```python
from build123d import *

# Parameters (mm, degrees)
BOSS_EXTRUDE1_OUTLINE_R = 7.5
BOSS_EXTRUDE1_DEPTH     = 30
SKETCH1_3_R             = 7.5
SKETCH1_3_R_2           = 5
BOSS_EXTRUDE2_DEPTH     = 5
FILLET1_R               = 10
CUT_EXTRUDE6_DEPTH      = 4
SKETCH5_3_R             = 2
CUT_EXTRUDE7_DEPTH      = 35
SKETCH10_R              = 1.5
CUT_EXTRUDE11_DEPTH     = 4
CUT_EXTRUDE12_START     = -2.5
SKETCH10_5_R            = 1.5
CUT_EXTRUDE12_DEPTH     = 2.5
CUT_EXTRUDE13_DEPTH     = 34


# Read off the part's stored shape, not the designer's step: Boss-Extrude1
with BuildPart() as part:
    # Boss-Extrude1 outline → Boss-Extrude1 (new body)
    with BuildSketch(Plane(origin=(0, 0, 0), x_dir=(1, 0, 0), z_dir=(0, 1, 0))):
        Polygon((-33.5, 13), (-33.5, -13), (-15, -13), (-15, -21.5), (-2, -21.5), (-2, -10.5), (2, -10.5), (2, -21.5), (15, -21.5), (15, -13), (33.5, -13), (33.5, 13), align=None)
        with Locations((-15, 0)):
            Circle(BOSS_EXTRUDE1_OUTLINE_R, mode=Mode.SUBTRACT)
        with Locations((15, 0)):
            Circle(BOSS_EXTRUDE1_OUTLINE_R, mode=Mode.SUBTRACT)
    extrude(amount=BOSS_EXTRUDE1_DEPTH)

    # Sketch1<3> → Boss-Extrude2 (add)
    # profile 1 of 2: a face of its own
    with BuildSketch(Plane(origin=(0, 0, 0), x_dir=(1, 0, 0), z_dir=(0, 1, 0))):
        with Locations(Location((-15, 0, 0), (0, 0, 270))):
            Circle(SKETCH1_3_R)
        with Locations(Location((-15, 0, 0), (0, 0, 270))):
            Circle(SKETCH1_3_R_2, mode=Mode.SUBTRACT)
    # profile 2 of 2: a face of its own
    with BuildSketch(Plane(origin=(0, 0, 0), x_dir=(1, 0, 0), z_dir=(0, 1, 0))):
        with Locations(Location((15, 0, 0), (0, 0, 270))):
            Circle(SKETCH1_3_R)
        with Locations(Location((15, 0, 0), (0, 0, 270))):
            Circle(SKETCH1_3_R_2, mode=Mode.SUBTRACT)
    extrude(amount=BOSS_EXTRUDE2_DEPTH)

    # Fillet1
    fillet1_edges = [part.edges().sort_by_distance(p)[0] for p in [
        (-33.5, 15, -13),
        (33.5, 15, -13),
        (33.5, 15, 13),
        (-33.5, 15, 13),
    ]]
    fillet(fillet1_edges, radius=FILLET1_R)

    # Sketch5 → Cut-Extrude6 (cut)
    with BuildSketch(Plane(origin=(15, 0, 0), x_dir=(0, 0, -1), z_dir=(1, 0, 0))):
        with BuildLine():
            Line((-20.75, 17.020725942), (-20.75, 15))
            Line((-20.75, 15), (-19.25, 15))
            ThreePointArc((-19.25, 15), (-17.25, 17), (-15.25, 15))
            Line((-15.25, 15), (-13.75, 15))
            Line((-13.75, 15), (-13.75, 17.020725942))
            Line((-13.75, 17.020725942), (-17.25, 19.041451884))
            Line((-17.25, 19.041451884), (-20.75, 17.020725942))
        make_face()
        with BuildLine():
            Line((-19.25, 15), (-20.75, 15))
            Line((-20.75, 15), (-20.75, 12.979274058))
            Line((-20.75, 12.979274058), (-17.25, 10.958548116))
            Line((-17.25, 10.958548116), (-13.75, 12.979274058))
            Line((-13.75, 12.979274058), (-13.75, 15))
            Line((-13.75, 15), (-15.25, 15))
            ThreePointArc((-15.25, 15), (-17.25, 13), (-19.25, 15))
        make_face()
    extrude(amount=-CUT_EXTRUDE6_DEPTH, mode=Mode.SUBTRACT)

    # Sketch5<3> → Cut-Extrude7 (cut)
    with BuildSketch(Plane(origin=(15, 0, 0), x_dir=(0, 0, -1), z_dir=(1, 0, 0))):
        with Locations((-17.25, 15)):
            Circle(SKETCH5_3_R)
    extrude(amount=-CUT_EXTRUDE7_DEPTH, mode=Mode.SUBTRACT)

    # Sketch10 → Cut-Extrude11 (cut)
    with BuildSketch(Plane(origin=(30.5, 0, 0), x_dir=(0, 0, -1), z_dir=(1, 0, 0))):
        with Locations((0, 22)):
            Circle(SKETCH10_R)
        with Locations((0, 8)):
            Circle(SKETCH10_R)
    cut_extrude11 = extrude(amount=CUT_EXTRUDE11_DEPTH, mode=Mode.SUBTRACT)

    # Sketch10<5> → Cut-Extrude12 (cut)
    # profile 1 of 5: a face of its own
    with BuildSketch(Plane(origin=(30.5, 0, 0), x_dir=(0, 0, -1), z_dir=(1, 0, 0)).offset(CUT_EXTRUDE12_START)):
        Polygon((-2.725, 30), (2.725, 30), (2.725, 23.573279484), (0, 25.146558967), (-2.725, 23.573279484), align=None)
    # profile 2 of 5: a face of its own
    with BuildSketch(Plane(origin=(30.5, 0, 0), x_dir=(0, 0, -1), z_dir=(1, 0, 0)).offset(CUT_EXTRUDE12_START)):
        Polygon((2.725, 20.426720516), (2.725, 23.573279484), (0, 25.146558967), (-2.725, 23.573279484), (-2.725, 20.426720516), (0, 18.853441033), align=None)
        with Locations((0, 22)):
            Circle(SKETCH10_5_R, mode=Mode.SUBTRACT)
    # profile 3 of 5: a face of its own
    with BuildSketch(Plane(origin=(30.5, 0, 0), x_dir=(0, 0, -1), z_dir=(1, 0, 0)).offset(CUT_EXTRUDE12_START)):
        with Locations((0, 22)):
            Circle(SKETCH10_5_R)
    # profile 4 of 5: a face of its own
    with BuildSketch(Plane(origin=(30.5, 0, 0), x_dir=(0, 0, -1), z_dir=(1, 0, 0)).offset(CUT_EXTRUDE12_START)):
        Polygon((-2.725, 6.426720516), (-2.725, 9.573279484), (0, 11.146558967), (2.725, 9.573279484), (2.725, 6.426720516), (2.725, 0), (-2.725, 0), align=None)
        with Locations((0, 8)):
            Circle(SKETCH10_5_R, mode=Mode.SUBTRACT)
    # profile 5 of 5: a face of its own
    with BuildSketch(Plane(origin=(30.5, 0, 0), x_dir=(0, 0, -1), z_dir=(1, 0, 0)).offset(CUT_EXTRUDE12_START)):
        with Locations((0, 8)):
            Circle(SKETCH10_5_R)
    cut_extrude12 = extrude(amount=CUT_EXTRUDE12_DEPTH, mode=Mode.SUBTRACT)

    # Sketch11 → Cut-Extrude13 (cut)
    with BuildSketch(Plane(origin=(0, 30, 0), x_dir=(1, 0, 0), z_dir=(0, 1, 0))):
        Polygon((28, 2.725), (28, 3.043492212), (25, 3.043492212), (25, -2.956507788), (28, -2.956507788), (28, -2.638015576), align=None)
    cut_extrude13 = extrude(amount=-CUT_EXTRUDE13_DEPTH, mode=Mode.SUBTRACT)

    # Mirror1: Cut-Extrude11, Cut-Extrude12, Cut-Extrude13 across plane
    add(cut_extrude11.mirror(Plane(origin=(0, 0, 0), x_dir=(0, 0, 1), z_dir=(1, 0, 0))), mode=Mode.SUBTRACT)
    add(cut_extrude12.mirror(Plane(origin=(0, 0, 0), x_dir=(0, 0, 1), z_dir=(1, 0, 0))), mode=Mode.SUBTRACT)
    add(cut_extrude13.mirror(Plane(origin=(0, 0, 0), x_dir=(0, 0, 1), z_dir=(1, 0, 0))), mode=Mode.SUBTRACT)


solid = part.part
```
Geometry check sheet. Reference: the model listing, model coordinates, mm. A direction names the side the tool comes from. Round coordinates to 2 decimals unless told otherwise and drop trailing zeros. Order: outer loops, then holes, each group sorted by start corner. A loop starts at its lowest first (then second) coordinate and runs counter-clockwise, first axis right, second up. Notation, with made-up numbers: M 68,52.5 L 122,52.5 A21 ccw 122,71.5 Z; hole C 80.25,72.25 d4. An arc over 180 degrees is marked long. Write item = value, one per line.
Q1. Scan lines: line 1 (X direction, y = 18, z = 0); line 2 (X direction, y = 10.5, z = 0); line 3 (Y direction, x = -31, z = 0). Record each from-to range of solid material in increasing order.
Answer block:
line_1 = -33.5 to -28, -25 to -22.5, -7.5 to 7.5, 22.5 to 25, 28 to 33.5
line_2 = -33.5 to -30.5, -25 to -22.5, -7.5 to 7.5, 22.5 to 25, 30.5 to 33.5
line_3 = 0 to 6.5, 9.5 to 20.5, 23.5 to 30
Q2. Section check A-A (y = 3). Give the number of separate pieces and of enclosed holes in the cut face, plus the area to 3 significant figures.
Answer block:
separate_pieces = 1
enclosed_holes = 4
area = 1,650 mm^2
Q3. Depth check by flat-ended pin: pin 1 Ø3 at (x, y) = (-28.5, 23.5) entering from -Z; pin 2 Ø2 at (y, z) = (8, 8.5) entering from +X; pin 3 Ø3.5 at (x, y) = (-27, 16) entering from +Z. Enter the tip coordinate at first touch or a pass-through.
Answer block:
pin_1 = -12.37
pin_2 = 32.43
pin_3 = 12.85
Q4. Section check B-B (z = 16.5). Enter the section's corners in (x, y).
Answer block:
outline = M -15,0 L -2,0 L -2,13.15 L -15,13.15 Z; M -15,16.85 L -2,16.85 L -2,30 L -15,30 Z; M 2,0 L 15,0 L 15,11.39 L 11,11.39 L 11,13.15 L 2,13.15 Z; M 2,16.85 L 11,16.85 L 11,18.61 L 15,18.61 L 15,30 L 2,30 Z
Q5. Release check for a two-part mould opening along Z. For faces 4 (the flat face through (-15, 15, 20)), 5 (the flat face through (13.03, 18.02, 15.48)), 6 (the cylindrical face through (-30.49, 15.21, -10.15)), 7 (the flat face through (-29, 25, 2.725)) record: released by +Z, released by -Z, zero draft, split by the parting line, or undercut.
Answer block:
face_4 = zero draft
face_5 = undercut
face_6 = released by -Z
face_7 = undercut
Q6. Set-up check for faces 1 (the cylindrical face through (-31.979, 6.536, 0.325)), 2 (the flat face through (-2, 15, 15)), 3 (the flat face through (-29.232, 10.371, -1.343)): record each of +Z, -Z, +X, -X, +Y, -Y from which the full face is reachable in a straight line by a thin tool's end or side.
Answer block:
face_1 = -X
face_2 = +Z, +Y, -Y
face_3 = -Y
Q7. Section check D-D (x = 26). Enter the section's corners in (y, z), plus the area to 3 significant figures.
Answer block:
outline = M 0,-12.68 L 30,-12.68 L 30,-3.04 L 0,-3.04 Z; M 0,2.96 L 30,2.96 L 30,12.68 L 0,12.68 Z
area = 581 mm^2
Q8. Section check C-C (x = 12.5). Enter the section's corners in (y, z), plus the area to 3 significant figures.
Answer block:
outline = M 0,-13 L 30,-13 L 30,-7.07 L 5,-7.07 L 5,-4.33 L 0,-4.33 Z; M 0,4.33 L 5,4.33 L 5,7.07 L 30,7.07 L 30,21.5 L 0,21.5 Z; hole M 10.96,17.25 L 12.98,13.75 L 17.02,13.75 L 19.04,17.25 L 17.02,20.75 L 12.98,20.75 Z
area = 596 mm^2
